The figure shows three views and two pictorial views of one solid part (mm, origin at its lowest corner). Answer the questions. A direction names the side the tool comes from. Round coordinates to 2 decimals unless told otherwise and drop trailing zeros. Write each loop counter-clockwise with the first axis right and the second up, starting at its lowest first coordinate (ties: lowest second). Pieces come first, ordered by that corner, then holes.
Item 1: A tool of negligible diameter and unlimited length cuts with its end or side. For the marked faces 4 and 5, from which of +Z, -Z, +X, -X, +Y, -Y can it reach the whole face along a straight path? Write none if from no direction.
Item 2: Find section B-B on y = 0.8. Give the vertices of the cut face in (x, z), then the cut area to 3 significant figures.
Item 3: This flat-tipped pin is pushed along its axis until it touches: pin 1 (3.5 mm diameter, centred on x = 3.937, z = 3.937, fed in from +Y). Where does it stop, or does it pass through?
Item 4: Find section A-A on x = 5. Give the number of separate pieces and of enclosed holes in the cut face.
Item 5: For a pull along X with two mould halves and no side action, classify the marked faces 1, 2 and 3 as +X half, -X half, draft (parallel to the pull), parting line (faces both ways), or undercut.
Item 6: Find the intervals of material crossed by probe 1 along X at (y, z) = (5.05, 4) (1 decimal); probe 2 along Z at (x, y) = (4, 2.7); probe 3 along X at (y, z) = (1.4, 6) (1 decimal), in increasing order.
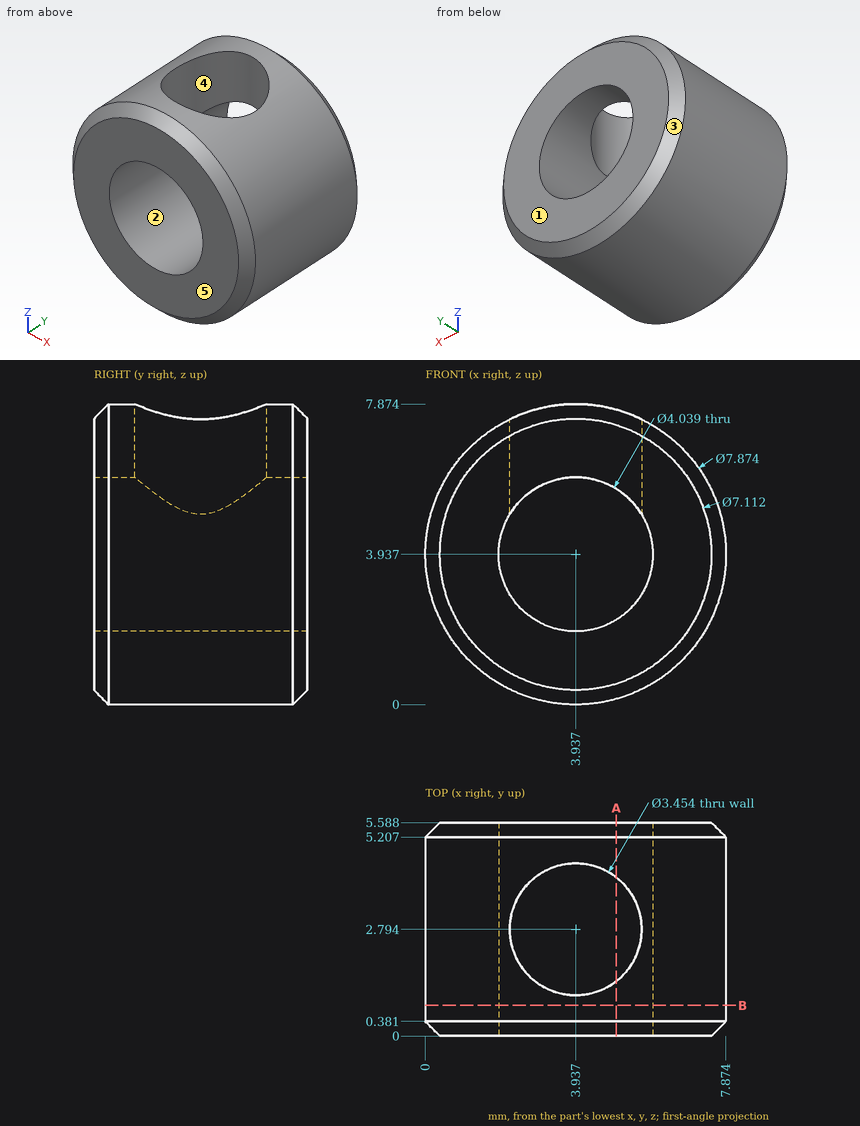
Check values:
1. face 4: +Z
1. face 5: +Z, -Z, +X, -X, -Y
2. outline: circle Ø7.87 at (3.94, 3.94); hole circle Ø4.04 at (3.94, 3.94)
2. area: 35.9 mm2
3. pin 1: passes through
4. separate pieces: 3
4. enclosed holes: 0
5. face 1: draft
5. face 2: undercut
5. face 3: parting line
6. probe 1: x = 0 to 1.9, 6 to 7.9
6. probe 2: z = 0 to 1.92
6. probe 3: x = 0.6 to 2.9, 5 to 7.3
